Part model, mm, in its own coordinate system. Face numbers are marked on the shaded views. A direction names the side the tool comes from. Round coordinates to 2 decimals unless told otherwise and drop trailing zeros. Write each loop counter-clockwise with the first axis right and the second up, starting at its lowest first coordinate (ties: lowest second). Pieces come first, ordered by that corner, then holes.
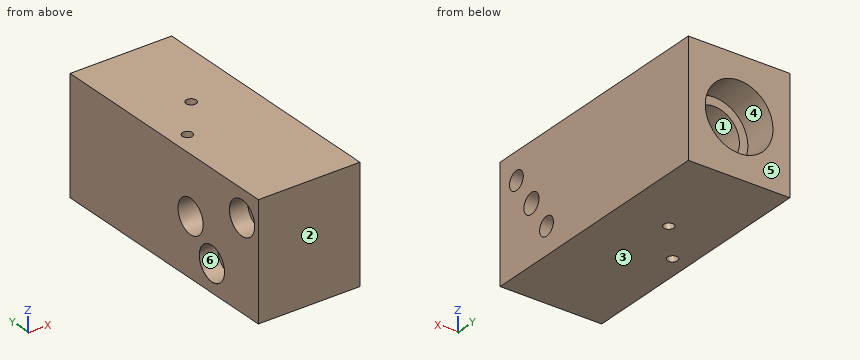
```python
from build123d import *

# Parameters (mm, degrees)
SCHIZZO1_W                    = 30
SCHIZZO1_H                    = 75
ESTRUSIONE_ESTRUSIONE1_DEPTH  = 17
FORO_6_0_6_1_D                = 6
FORO_6_0_6_1_DEPTH            = 20
FORO_6_0_6_1_TIP              = 1.802581857
SCHIZZO6_R                    = 10
TAGLIO_ESTRUSIONE1_DEPTH      = 10
SCHIZZO7_R                    = 7.5
TAGLIO_ESTRUSIONE2_DEPTH      = 20
SCHIZZO8_R                    = 5
TAGLIO_ESTRUSIONE3_DEPTH      = 25
TAGLIO_ESTRUSIONE4_REACH      = 66.915
TAGLIO_ESTRUSIONE4_END_RADIUS = 3
SCHIZZO9_R                    = 1.5
TAGLIO_ESTRUSIONE5_REACH      = 84.547
TAGLIO_ESTRUSIONE5_END_RADIUS = 5
SCHIZZO10_R                   = 5
TAGLIO_ESTRUSIONE5_DRAFT      = -1
TAGLIO_ESTRUSIONE6_REACH      = 89.641
SCHIZZO11_R                   = 1.5


# Read off the part's stored shape, not the designer's step: Foro lamato per Vite M5 a testa cilindrica-1
with BuildPart() as part:
    # Schizzo1 → Estrusione-Estrusione1 (new, symmetric)
    with BuildSketch(Plane.XY):
        with Locations((15, 37.5)):
            Rectangle(SCHIZZO1_W, SCHIZZO1_H)
    extrude(amount=ESTRUSIONE_ESTRUSIONE1_DEPTH, both=True)

    # Foro Ø6.0 (6)-1
    with Locations(Plane(origin=(30, 12.5, 0), x_dir=(0, 0, 1), z_dir=(1, 0, 0))):
        with Locations((0, 0)):
            Hole(FORO_6_0_6_1_D / 2, depth=FORO_6_0_6_1_DEPTH)
            with Locations((0, 0, -(FORO_6_0_6_1_DEPTH + FORO_6_0_6_1_TIP / 2))):  # 118° drill point
                Cone(0, FORO_6_0_6_1_D / 2, FORO_6_0_6_1_TIP, mode=Mode.SUBTRACT)

    # Foro lamato per Vite M5 a testa cili 2 → Foro lamato per Vite M5 a testa cilindrica-1 (revolve, cut)
    with BuildSketch(Plane(origin=(0, 6.5, 9), x_dir=(0, 1, 0), z_dir=(0, 0, -1))):
        Polygon((2.75, 5.4), (2.75, 30), (0, 30), (0, 0), (5.025, 0), (5, 0.025), (5, 5.4), align=None)
    revolve(axis=Axis((0, 6.5, 9), (1, 0, 0)), mode=Mode.SUBTRACT)

    # Foro lamato per Vite M5 a testa cili 3 o → Foro lamato per Vite M5 a testa cili 3 (revolve, cut)
    with BuildSketch(Plane(origin=(0, 18.5, -9), x_dir=(0, 1, 0), z_dir=(0, 0, -1))):
        Polygon((0, 0), (5.025, 0), (5, 0.025), (5, 5.4), (2.75, 5.4), (2.75, 30), (0, 30), align=None)
    revolve(axis=Axis((0, 18.5, -9), (1, 0, 0)), mode=Mode.SUBTRACT)

    # Schizzo6 → Taglio-Estrusione1 (cut)
    with BuildSketch(Plane(origin=(0, 75, 0), x_dir=(1, 0, 0), z_dir=(0, 1, 0))):
        with Locations(Location((15, 0, 0), (0, 0, 270))):
            Circle(SCHIZZO6_R)
    extrude(amount=-TAGLIO_ESTRUSIONE1_DEPTH, mode=Mode.SUBTRACT)

    # Schizzo7 → Taglio-Estrusione2 (cut)
    with BuildSketch(Plane(origin=(0, 65, 0), x_dir=(1, 0, 0), z_dir=(0, 1, 0))):
        with Locations(Location((15, 0, 0), (0, 0, 270))):
            Circle(SCHIZZO7_R)
    extrude(amount=-TAGLIO_ESTRUSIONE2_DEPTH, mode=Mode.SUBTRACT)

    # Schizzo8 → Taglio-Estrusione3 (cut)
    with BuildSketch(Plane(origin=(0, 45, 0), x_dir=(1, 0, 0), z_dir=(0, 1, 0))):
        with Locations(Location((15, 0, 0), (0, 0, 270))):
            Circle(SCHIZZO8_R)
    extrude(amount=-TAGLIO_ESTRUSIONE3_DEPTH, mode=Mode.SUBTRACT)

    # Taglio-Estrusione4: up to this cylinder (the profile starts outside it)
    taglio_estrusione4_end = Plane(origin=(15, 12.5, 0), z_dir=(1, 0, 0)) * Cylinder(TAGLIO_ESTRUSIONE4_END_RADIUS, 140.83, mode=Mode.PRIVATE)
    # Schizzo9 → Taglio-Estrusione4 (cut, up to the surface)
    with BuildSketch(Plane(origin=(0, 20, 0), x_dir=(1, 0, 0), z_dir=(0, 1, 0)), mode=Mode.PRIVATE) as taglio_estrusione4_sk1:
        with Locations(Location((15, 0, 0), (0, 0, 270))):
            Circle(SCHIZZO9_R)
    taglio_estrusione4_tool1 = extrude(taglio_estrusione4_sk1.sketch, amount=-TAGLIO_ESTRUSIONE4_REACH, mode=Mode.PRIVATE) - taglio_estrusione4_end
    add(taglio_estrusione4_tool1.solids().sort_by_distance((15, 20, 0))[0], mode=Mode.SUBTRACT)

    # Taglio-Estrusione5: up to this cylinder (the profile starts outside it)
    taglio_estrusione5_end = Plane(origin=(15, 27, 0), z_dir=(0, 1, 0)) * Cylinder(TAGLIO_ESTRUSIONE5_END_RADIUS, 180.094, mode=Mode.PRIVATE)



with BuildPart() as taglio_estrusione5_long_prism_1:
    # Schizzo10 → Taglio-Estrusione5 (the long prism of profile 1, to be tilted and cut off)
    with BuildSketch(Plane.ZY):
        with Locations((0, 27)):
            Circle(SCHIZZO10_R)
    extrude(amount=-TAGLIO_ESTRUSIONE5_REACH)
    taglio_estrusione5_tool1_sides = [taglio_estrusione5_long_prism_1.faces().sort_by_distance(p)[0] for p in [
        (42.2735, 27, -5),
    ]]
    draft(taglio_estrusione5_tool1_sides, Plane.ZY, TAGLIO_ESTRUSIONE5_DRAFT)  # the draft: side faces tilted about the start plane


with BuildPart() as part_1:
    add(part.part)
    taglio_estrusione5_tool1 = taglio_estrusione5_long_prism_1.part - taglio_estrusione5_end
    add(taglio_estrusione5_tool1.solids().sort_by_distance((0, 27, 0))[0], mode=Mode.SUBTRACT)

    # Taglio-Estrusione6: up to this face of the body (flat: up to its plane)
    taglio_estrusione6_end = Plane(part_1.part.faces().sort_by_distance((15, 37.5, -17))[0])
    # Schizzo11 → Taglio-Estrusione6 (cut, up to the picked face)
    with BuildSketch(Plane.XY.offset(17), mode=Mode.PRIVATE) as taglio_estrusione6_sk1:
        with Locations((5, 35)):
            Circle(SCHIZZO11_R)
    taglio_estrusione6_tool1 = split(extrude(taglio_estrusione6_sk1.sketch, amount=-TAGLIO_ESTRUSIONE6_REACH, mode=Mode.PRIVATE), bisect_by=taglio_estrusione6_end, keep=Keep.BOTH, mode=Mode.PRIVATE)
    # Schizzo11 → Taglio-Estrusione6 (cut, up to the picked face)
    with BuildSketch(Plane.XY.offset(17), mode=Mode.PRIVATE) as taglio_estrusione6_sk2:
        with Locations((15, 47)):
            Circle(SCHIZZO11_R)
    taglio_estrusione6_tool2 = split(extrude(taglio_estrusione6_sk2.sketch, amount=-TAGLIO_ESTRUSIONE6_REACH, mode=Mode.PRIVATE), bisect_by=taglio_estrusione6_end, keep=Keep.BOTH, mode=Mode.PRIVATE)
    add(taglio_estrusione6_tool1.solids().sort_by(Axis((5, 35, 17), (0, 0, -1)))[0], mode=Mode.SUBTRACT)
    add(taglio_estrusione6_tool2.solids().sort_by(Axis((15, 47, 17), (0, 0, -1)))[0], mode=Mode.SUBTRACT)


solid = part_1.part
```
Q1. Wall check: L1, parallel to Z at x = 21, y = 6.5; L2, parallel to Z at x = 15, y = 17; L3, parallel to X at y = 48, z = 5.5. Give the ranges that are in metal, low to high.
Values follow:
L1: z = -17 to 6.25, 11.75 to 17
L2: z = -17 to -11.3, -6.7 to -1.5, 1.5 to 17
L3: x = 0 to 9.9, 20.1 to 30
Q2. Mould opens along Z. For the marked faces 1, 2 and 3 say: +Z half, -Z half, draft (parallel to the pull), parting line (faces both ways), or undercut.
Values follow:
face 1: undercut
face 2: draft
face 3: -Z half
Q3. Which spindle directions (+Z, -Z, +X, -X, +Y, -Y) get a long thin tool onto all of the face, cutting with end or side? Do the marked faces 4, 5 and 6. Say none if no direction does.
Values follow:
face 4: +Y
face 5: +Z, -Z, +X, -X, +Y
face 6: -X
Q4. Cut at A-A on y = 35. Write the cut outline in (x, z).
Values follow:
outline: (0, -17) - (3.5, -17) - (3.5, 17) - (0, 17) - close; (6.5, -17) - (30, -17) - (30, 17) - (6.5, 17) - close; hole circle Ø10 at (15, 0)
Q5. Cut at D-D on x = 28. Write the cut outline in (y, z), plus the area to 3 significant figures.
Values follow:
outline: (0, -17) - (75, -17) - (75, 17) - (0, 17) - close; hole circle Ø5.5 at (6.5, 9); hole circle Ø6 at (12.5, 0); hole circle Ø5.5 at (18.5, -9)
area: 2,470 mm2
Q6. Drop flat-ended pins along their axis: pin 1 (1 mm diameter, centred on x = 16, z = 8, fed in from +Y); pin 2 (6 mm diameter, centred on x = 13, z = -2, fed in from +Y); pin 3 (4 mm diameter, centred on x = 15, z = 0, fed in from +Y). Give the stop position or say it passes through.
Values follow:
pin 1: stops at y = 65
pin 2: stops at y = 45
pin 3: stops at y = 20
Q7. Cut at C-C on y = 67. Write the cut outline in (x, z).
Values follow:
outline: (0, -17) - (30, -17) - (30, 17) - (0, 17) - close; hole circle Ø20 at (15, 0)
Q8. Cut at B-B on x = 21. Write the cut outline in (y, z), plus the area to 3 significant figures.
Values follow:
outline: (0, -17) - (75, -17) - (75, -8) - (65, -8) - (65, -4.5) - (45, -4.5) - (45, 4.5) - (65, 4.5) - (65, 8) - (75, 8) - (75, 17) - (0, 17) - close; hole circle Ø5.5 at (6.5, 9); hole circle Ø6 at (12.5, 0); hole circle Ø5.5 at (18.5, -9)
area: 2,130 mm2
